Could you check a few things on this model? Use its own coordinates, in mm. A direction names the side the tool comes from. Coordinates: 2 decimals unless noted, no trailing zeros. Write each loop counter-clockwise with the first axis right and the second up, starting at its lowest first coordinate (ties: lowest second). Pieces come first, ordered by that corner, then holes.
Item 1: For P1, Ø12, axis at x = 40, y = 42.5, coming from the -Z side; P2, Ø3.5, axis at y = 50, z = 2, coming from the +X side; P3, Ø1.5, axis at x = -1, y = 44.5, coming from the +Z side; P4, Ø3.5, axis at x = 53, z = 2.5, coming from the +Y side, each with a flat end and sliding along its axis, tell me the tip position at first contact or that it passes through.
Item 2: I want a section at A-A on z = 4.5. Please give me the cut outline in (x, y).
Item 3: I want a section at D-D on x = 26. Please give me the cut outline in (y, z).
Item 4: I want a section at B-B on y = 49.5. Please give me the cut outline in (x, z), then the cut area to 3 significant figures.
Item 5: Thinking about a two-plate mould opening in Y: for faces 1 (the flat face through (25, -2.5, 1)), 2 (the cylindrical face through (-1.5, -0.07, 2.96)), 3 (the flat face through (47.5, 49, 3)), which applies, +Y half, -Y half, draft (parallel to the pull), parting line (faces both ways), or undercut?
Item 6: Which directions (+Z, -Z, +X, -X, +Y, -Y) give clear straight access to the entire face, cutting with the end or side of a thin tool? Please do faces 4 (the cylindrical face through (1.787, 43.252, 3.972)), 5 (the flat face through (-2.5, 22, 1)), 6 (the flat face through (2.5, -4, 3)), 7 (the flat face through (25, 47.5, 1)).
Item 7: If I drill on probe 1 along X at (y, z) = (45, 4.25); probe 2 along Y at (x, z) = (0, 1.6); probe 3 along Y at (x, z) = (50, 4.2), over which ranges is the centre line in solid material (lowest first)?
Item 8: I want a section at C-C on y = 34.5. Please give me the cut outline in (x, z), then the cut area to 3 significant figures.
Autodesk Fusion 360 part; units mm, degrees
sketch "Sketch1" plane through (0, 0, 0) normal (0, 0, 1) x (1, 0, 0)
  line L0 (0, 0) -> (60, 0)
  line L1 (60, 0) -> (60, 60)
  line L2 (60, 60) -> (0, 60)
  line L3 (0, 60) -> (0, 0)
  line L4 (2, 2) -> (58, 2)
  line L5 (58, 2) -> (58, 58)
  line L6 (58, 58) -> (2, 58)
  line L7 (2, 58) -> (2, 2)
  dimension "d1" = 60
  dimension "d2" = 60
  dimension "d3" = 56
  dimension "d4" = 56
sketch "Sketch2" plane through (0, 0, 2) normal (0, 0, 1) x (-1, 0, 0)
  line L0 (-2, -2) -> (-4.5, -2)
  line L1 (-4.5, -2) -> (-4.5, -5)
  line L2 (-4.5, -5) -> (-2, -5)
  line L3 (-2, -5) -> (-2, -2)
  line L4 (-2, -58) -> (-4.5, -58)
  line L5 (-4.5, -58) -> (-4.5, -55)
  line L6 (-4.5, -55) -> (-2, -55)
  line L7 (-2, -55) -> (-2, -58)
  line L8 (-58, -58) -> (-49.5, -58)
  line L9 (-49.5, -58) -> (-49.5, -55)
  line L10 (-49.5, -55) -> (-58, -55)
  line L11 (-58, -55) -> (-58, -58)
  line L12 (-58, -2) -> (-49.5, -2)
  line L13 (-49.5, -2) -> (-49.5, -5)
  line L14 (-49.5, -5) -> (-58, -5)
  line L15 (-58, -5) -> (-58, -2)
  circle A0 centre (-4.5, -55) radius 1
  circle A1 centre (-49.5, -55) radius 1
  circle A2 centre (-4.5, -5) radius 1
  circle A3 centre (-49.5, -5) radius 1
  line L16 (-2, -58) -> (-2, -2)
  line L17 (-2, -2) -> (-58, -2)
  line L18 (-58, -2) -> (-58, -58)
  line L19 (-58, -58) -> (-2, -58)
  dimension "d9" = 2.5
  dimension "d10" = 3
  dimension "d11" = 2.5
  dimension "d12" = 3
  dimension "d13" = 8.5
  dimension "d14" = 3
  dimension "d15" = 8.5
  dimension "d16" = 3
  dimension "d17" = 2
  dimension "d18" = 2
  dimension "d19" = 2
  dimension "d20" = 2
sketch "Sketch3" plane through (0, 0, 0) normal (0, 0, 1) x (1, 0, 0)
  circle A0 centre (0, 45) radius 1.5
  circle A1 centre (50, 45) radius 1.5
  circle A2 centre (50, 0) radius 1.5
  circle A3 centre (0, 0) radius 1.5
  line L0 (0, -2.5) -> (50, -2.5)
  line L1 (52.5, 0) -> (52.5, 45)
  line L2 (-2.5, 0.0027) -> (-2.5, 45)
  line L3 (0.0001, 47.5) -> (50, 47.5)
  circle A4 centre (0, 45) radius 7.5
  circle A5 centre (0, 0) radius 7.5
  circle A6 centre (50, 45) radius 7.5
  circle A7 centre (50, 0) radius 7.5
  line L4 (0, 42.5) -> (-7.0711, 42.5)
  line L5 (2.5, 45) -> (2.5, 52.0711)
  line L6 (47.5, 45) -> (47.5, 52.0711)
  line L7 (50, 42.5) -> (57.0711, 42.5)
  line L8 (50, 2.5) -> (57.0711, 2.5)
  line L9 (47.5, 0) -> (47.5, -7.0711)
  line L10 (0, 2.5) -> (-7.0711, 2.5)
  line L11 (2.5, 0) -> (2.5, -7.0711)
  arc A8 (0, 42.5) -> (2.5, 45) centre (0, 45) ccw
  arc A9 (0.0001, 47.5) -> (-2.5, 45) centre (0, 45) ccw
  line L12 (0, 45) -> (0, 43.5)
  line L13 (1.5, 45) -> (0, 45)
  arc A10 (47.5, 45) -> (50, 42.5) centre (50, 45) ccw
  arc A11 (52.5, 45) -> (50, 47.5) centre (50, 45) ccw
  line L14 (50, 43.5) -> (50, 45)
  line L15 (50, 45) -> (48.5, 45)
  line L16 (47.5, 45) -> (2.5, 45)
  arc A12 (50, 2.5) -> (47.5, 0) centre (50, 0) ccw
  arc A13 (50, -2.5) -> (52.5, 0) centre (50, 0) ccw
  line L17 (48.5, 0) -> (50, 0)
  line L18 (50, 0) -> (50, 1.5)
  line L19 (50, 2.5) -> (50, 42.5)
  arc A14 (-2.5, 0.0027) -> (0, -2.5) centre (0, 0) ccw
  arc A15 (2.5, 0) -> (0, 2.5) centre (0, 0) ccw
  line L20 (0, 0) -> (1.5, 0)
  line L21 (2.5, 0) -> (47.5, 0)
  line L22 (0, 42.5) -> (0, 2.5)
  line L23 (0, 1.5) -> (0, 0)
  dimension "d23" = 50
  dimension "d24" = 45
  dimension "d25" = 3
  dimension "d26" = 3
  dimension "d27" = 3
  dimension "d28" = 3
  dimension "d29" = 5
  dimension "d30" = 5
  dimension "d31" = 5
  dimension "d32" = 5
  dimension "d37" = 15
  dimension "d38" = 15
  dimension "d39" = 15
  dimension "d40" = 15
extrude "Extrude6" add sketch "Sketch3" along normal blind 7 contours L0 L2 A5 L10 L11 A14 | L0 L1 A7 L8 L9 A13 | L2 L3 A4 L4 L5 A9 | L1 L3 A6 L6 L7 A11 makes body 1 at (48.1731, 52.2741, 2.3333) makes body 2 at (48.8622, -7.4132, 4.6667) makes body 3 at (-7.4132, 43.8622, 2.3333) makes body 4 at (2.1658, -7.1805, 4.6667)
extrude "Extrude7" add sketch "Sketch3" along normal blind 2 separate body contours L0 A5 L11 L21 | L0 A5 A7 L21 | A5 A15 L21 L22 | L2 A5 L10 L22 | L0 A7 L9 L21 | A4 A5 A6 A7 L16 L19 L21 L22 | L2 A4 A5 L22 | A7 A12 L19 L21 | L2 A4 L4 L22 | L1 A6 A7 L19 | L1 A7 L8 L19 | A4 A8 L16 L22 | L1 A6 L7 L19 | A6 A10 L16 L19 | L3 A4 L5 L16 | L3 A4 A6 L16 | L3 A6 L6 L16 makes body 5
extrude "Extrude8" add sketch "Sketch3" along normal blind 6 contours L0 L2 L10 L11 A14 A15 | L0 L1 L8 L9 A12 A13 | L2 L3 L4 L5 A8 A9 | L1 L3 L6 L7 A10 A11 bodies 1 2 3 4 5
Response values:
1. P1: stops at z = 0
1. P2: stops at x = 56.76
1. P3: stops at z = 6
1. P4: stops at y = 52.4
2. outline: (-7.07, 2.5) arc R7.5 ccw to (2.5, -7.07) - (2.5, 0) arc R2.5 ccw to (0, 2.5) - close; (-7.07, 42.5) - (0, 42.5) arc R2.5 ccw to (2.5, 45) - (2.5, 52.07) arc R7.5 ccw to start; (47.5, -7.07) arc R7.5 ccw to (57.07, 2.5) - (50, 2.5) arc R2.5 ccw to (47.5, 0) - close; (47.5, 45) arc R2.5 ccw to (50, 42.5) - (57.07, 42.5) arc R7.5 ccw to (47.5, 52.07) - close; hole circle Ø3 at (0, 0); hole circle Ø3 at (0, 45); hole circle Ø3 at (50, 0); hole circle Ø3 at (50, 45)
3. outline: (-2.5, 0) - (47.5, 0) - (47.5, 2) - (-2.5, 2) - close
4. outline: (-6, 0) - (2.5, 0) - (2.5, 7) - (-6, 7) - close; (47.5, 0) - (56, 0) - (56, 7) - (47.5, 7) - close
4. area: 119 mm2
5. face 1: -Y half
5. face 2: undercut
5. face 3: draft
6. face 4: +Z
6. face 5: +Z, -Z, -X
6. face 6: +Z, -Y
6. face 7: +Z, -Z, +Y
7. probe 1: x = -7.5 to -1.5, 1.5 to 2.5, 47.5 to 48.5, 51.5 to 57.5
7. probe 2: y = -7.5 to -1.5, 1.5 to 43.5, 46.5 to 52.5
7. probe 3: y = -7.5 to -1.5, 1.5 to 2.5, 42.5 to 43.5, 46.5 to 52.5
8. outline: (-2.5, 0) - (52.5, 0) - (52.5, 2) - (-2.5, 2) - close
8. area: 110 mm2
